```python
from build123d import *

# Parameters (mm, degrees)
F1_DEPTH    = 40
F2_R        = 1
F3_T1_DEPTH = 168.4279953904


# Not quite as in the source:
# - a fillet or chamfer that OpenCascade refuses, or shapes differently, is made with other operations: its cross-section is extruded or revolved along the edge and cut away or added


with BuildPart() as f1:
    # F0 (on Top) → F1 (new body)
    with BuildSketch(Plane.XY):
        with BuildLine():
            Line((0, 2.15), (0, 8.41))
            Line((0, 8.41), (-6.1, 8.41))
            Line((-6.1, 8.41), (-6.1, -1.59))
            ThreePointArc((-6.1, -1.59), (-4.7073896383, -4.2954889128), (-2.25, -6.09))
            Line((-2.25, -6.09), (0, -6.09))
            Line((0, -6.09), (0, -2.15))
            ThreePointArc((0, -2.15), (-2.15, 0), (0, 2.15))
        make_face()
        with BuildLine():
            Line((6.1, -1.59), (6.1, 8.41))
            Line((6.1, 8.41), (0, 8.41))
            Line((0, 8.41), (0, 2.15))
            ThreePointArc((0, 2.15), (1.5202795796, 1.5202795796), (2.15, 0))
            ThreePointArc((2.15, 0), (1.5202795796, -1.5202795796), (0, -2.15))
            Line((0, -2.15), (0, -6.09))
            Line((0, -6.09), (2.25, -6.09))
            ThreePointArc((2.25, -6.09), (4.7073896383, -4.2954889128), (6.1, -1.59))
        make_face()
        with BuildLine():
            Line((33.9, 8.41), (6.1, 8.41))
            Line((6.1, 8.41), (6.1, -1.59))
            ThreePointArc((6.1, -1.59), (4.7073896383, -4.2954889128), (2.25, -6.09))
            Line((2.25, -6.09), (33.9, -6.09))
            Line((33.9, -6.09), (33.9, 8.41))
        make_face()
    extrude(amount=F1_DEPTH)

    # F2
    f2_edges = [f1.edges().sort_by_distance(p)[0] for p in [
        (-2.25, -6.09, 20),
    ]]
    fillet(f2_edges, radius=F2_R)

    # F3: fillet of radius 30 on 1 edges, made by hand

    # F3_s2 → F3_t1 (cut)
    with BuildSketch(Plane.XY.offset(-64.2139976952)):
        with BuildLine():
            ThreePointArc((8.2144009219, -6.09), (22.9622821257, -2.2147009552), (33.9, 8.41))
            Line((33.9, 8.41), (33.9, -6.09))
            Line((33.9, -6.09), (8.2144009219, -6.09))
        make_face()
    extrude(amount=F3_T1_DEPTH, mode=Mode.SUBTRACT)


solid = f1.part
```
Source: CAD feature listing. Evaluate the final solid. Frame: model axes, mm. Give positions to 0.01 mm unless a question says otherwise; leave off trailing zeros. Write each loop counter-clockwise with the first axis right and the second up, starting at its lowest first coordinate (ties: lowest second). Pieces come first, ordered by that corner, then holes.
1. Material intervals for line 1 along X through (y, z) = (0.5, 11.5); line 2 along X through (y, z) = (0.75, 21); line 3 along X through (y, z) = (2.5, 36), sorted ascending.
2. Section query C-C (x = -4). Return the cut outline in (y, z).
3. Section query D-D (y = 6.5). Return the cut outline in (x, z), then the cut area to 3 significant figures.
4. First-contact query: pin 1 (12 mm diameter, centred on x = 10, z = 22, fed in from -Y); pin 2 (3 mm diameter, centred on y = -1, z = 30.5, fed in from +X). Flat tips, straight axial feed; report the tip coordinate or a pass-through.
5. Section query B-B (z = 3.5). Return the cut outline in (x, y).
6. Section query A-A (y = 1). Return the cut outline in (x, z), then the cut area to 3 significant figures.
Output values:
1. line 1: x = -6.1 to -2.09, 2.09 to 26.98
1. line 2: x = -6.1 to -2.01, 2.01 to 27.28
1. line 3: x = -6.1 to 29.23
2. outline: (-5.01, 0) - (8.41, 0) - (8.41, 40) - (-5.01, 40) - close
3. outline: (-6.1, 0) - (32.65, 0) - (32.65, 40) - (-6.1, 40) - close
3. area: 1,550 mm2
4. pin 1: stops at y = -6.09
4. pin 2: stops at x = 26.98
5. outline: (-6.1, -1.59) arc R6.61 ccw to (-2.46, -6) arc R1 ccw to (-2.04, -6.09) - (8.21, -6.09) arc R30 ccw to (33.9, 8.41) - (-6.1, 8.41) - close; hole circle Ø4.3 at (0, 0)
6. outline: (-6.1, 0) - (-1.9, 0) - (-1.9, 40) - (-6.1, 40) - close; (1.9, 0) - (27.58, 0) - (27.58, 40) - (1.9, 40) - close
6. area: 1,200 mm2
